Autodesk Inventor part; units mm, degrees
ref_plane "YZ Plane" through (0, 0, 0) normal (1, 0, 0) x (0, 1, 0)
ref_plane "XZ Plane" through (0, 0, 0) normal (0, 1, 0) x (-1, 0, 0)
ref_plane "XY Plane" through (0, 0, 0) normal (0, 0, 1) x (1, 0, 0)
sketch "Sketch17" plane through (0, 0, 0) normal (0, 0, 1) x (1, 0, 0)
  line L0 (-3.0888, 0.15) -> (-1.6743, 2.6)
  line L1 (-1.4145, 2.75) -> (1.4145, 2.75)
  line L2 (1.6743, 2.6) -> (3.0888, 0.15)
  line L3 (3.0888, -0.15) -> (1.6743, -2.6)
  line L4 (1.4145, -2.75) -> (-1.4145, -2.75)
  line L5 (-1.6743, -2.6) -> (-3.0888, -0.15)
  circle A0 centre (0, 0) radius 1.5
  arc A1 (-1.4145, 2.75) -> (-1.6743, 2.6) centre (-1.4145, 2.45) ccw
  arc A2 (1.6743, 2.6) -> (1.4145, 2.75) centre (1.4145, 2.45) ccw
  arc A3 (3.0888, -0.15) -> (3.0888, 0.15) centre (2.829, 0) ccw
  arc A4 (1.4145, -2.75) -> (1.6743, -2.6) centre (1.4145, -2.45) ccw
  arc A5 (-1.6743, -2.6) -> (-1.4145, -2.75) centre (-1.4145, -2.45) ccw
  arc A6 (-3.0888, 0.15) -> (-3.0888, -0.15) centre (-2.829, 0) ccw
  point P0 (-3.1754, 0)
  point P1 (-1.5877, 2.75)
  point P2 (1.5877, 2.75)
  point P3 (3.1754, 0)
  point P4 (1.5877, -2.75)
  point P5 (-1.5877, -2.75)
  dimension "d103" = 5.5
  dimension "d104" = 3
  dimension "d105" = 0.3
extrude "Extrusion14" add sketch "Sketch17" along normal blind 2.4
sketch "Sketch18" plane through (0, 0, 0) normal (0, 1, 0) x (-1, 0, 0)
  line L0 (-3.0888, 2.4) -> (-1.6743, 2.4)
  line L1 (-1.6743, 0) -> (-1.6743, 2.4)
  line L2 (-3.0888, 0) -> (-1.6743, 0)
  line L3 (-3.0888, 0) -> (-3.0888, 2.4)
  line L4 (-1.5, 2.4) -> (1.5, 2.4)
  line L5 (1.5, 0) -> (-1.5, 0)
  line L6 (1.6743, 2.4) -> (3.0888, 2.4)
  line L7 (3.0888, 0) -> (3.0888, 2.4)
  line L8 (1.6743, 0) -> (3.0888, 0)
  line L9 (1.6743, 0) -> (1.6743, 2.4)
  line L10 (0, 2.4) -> (0, 4.8692)
  line L11 (0, 4.8692) -> (0, -2.1161)
  line L12 (1.4145, 0) -> (1.6743, 0)
  line L13 (1.4145, 2.4) -> (1.6743, 2.4)
  line L14 (1.6743, 0) -> (1.6743, 2.4)
  line L15 (1.4145, 0) -> (1.6743, 0)
  line L16 (1.4145, 0) -> (1.4145, 2.4)
  line L17 (2.5888, 3.8507) -> (2.5888, -1.604) construction
  line L18 (4.0837, 1.5369) -> (4.0837, 3.518)
  line L19 (4.0837, 3.518) -> (2.5888, 3.518)
  line L20 (2.5888, 2.4) -> (2.5888, 3.518)
  line L21 (2.5888, 0) -> (4.2933, 0.9841)
  line L22 (4.2933, 0.9841) -> (4.2933, -0.6301)
  line L23 (4.2933, -0.6301) -> (2.5888, -0.6301)
  line L24 (2.5888, -0.6301) -> (2.5888, 0)
  line L25 (2.5888, 2.4) -> (4.0837, 1.5369)
  dimension "d110" = 30
  dimension "d111" = 30
  dimension "d115" = 0.5
revolve "Revolution1" cut sketch "Sketch18" angle 360 about axis through (0, 0, 4.8692) along (0, 0, -1) contours L20 L19 L18 L25 L7 L6 | L6 L7 L25 | L21 L7 L8 | L8 L7 L21 L22 L23 L24
thread "Thread3"
chamfer "Chaflán9" distance 0.2 angle 45 1 edges at (-1.5, 0, 2.4)
chamfer "Chaflán10" distance 0.2 angle 45 1 edges at (-1.5, 0, 0)
properties part number "CF-TCA-0001"
Geometry check sheet. Reference: the model listing, model coordinates, mm. Coordinates: 2 decimals unless noted, no trailing zeros. Order: outer loops, then holes, each group sorted by start corner. A loop starts at its lowest first (then second) coordinate and runs counter-clockwise, first axis right, second up.
Q1. Thickness scan on probe 1 along Y at (x, z) = (0, 1.4); probe 2 along Y at (x, z) = (-0.5, 1.85); probe 3 along X at (y, z) = (-0.7, 1.9). Record the ranges inside material, lowest first.
Reply:
probe 1: y = -2.75 to -1.5, 1.5 to 2.75
probe 2: y = -2.75 to -1.41, 1.41 to 2.75
probe 3: x = -2.77 to -1.33, 1.33 to 2.77
Q2. Draft check along X on faces 1 (the face through (2.39, -1.36, 1.18)), 2 (the face through (-1.5, -0.07, 1.19)), 3 (the face through (0, 2.75, 1)), 4 (the face through (-2.372, -1.392, 1.185)). Enter one of: released by +X, released by -X, zero draft, split by the parting line, or undercut.
Reply:
face 1: released by +X
face 2: undercut
face 3: zero draft
face 4: released by -X
Q3. Sectioned sample at A-A on x = 0. Record the cut outline in (y, z), and give its area (3 significant figures).
Reply:
outline: (-2.75, 0.09) - (-2.59, 0) - (-1.7, 0) - (-1.5, 0.2) - (-1.5, 2.2) - (-1.7, 2.4) - (-2.59, 2.4) - (-2.75, 2.31) - close; (1.5, 0.2) - (1.7, 0) - (2.59, 0) - (2.75, 0.09) - (2.75, 2.31) - (2.59, 2.4) - (1.7, 2.4) - (1.5, 2.2) - close
area: 5.89 mm2
Q4. Sectioned sample at B-B on z = 1.25. Record the cut outline in (x, y).
Reply:
outline: (-3.09, -0.15) - (-1.67, -2.6) arc R0.3 ccw to (-1.41, -2.75) - (1.41, -2.75) arc R0.3 ccw to (1.67, -2.6) - (3.09, -0.15) arc R0.3 ccw to (3.09, 0.15) - (1.67, 2.6) arc R0.3 ccw to (1.41, 2.75) - (-1.41, 2.75) arc R0.3 ccw to (-1.67, 2.6) - (-3.09, 0.15) arc R0.3 ccw to start; hole circle Ø3 at (0, 0)
Q5. Sectioned sample at C-C on y = 0. Record the cut outline in (x, z).
Reply:
outline: (-3.13, 0.31) - (-2.59, 0) - (-1.7, 0) - (-1.5, 0.2) - (-1.5, 2.2) - (-1.7, 2.4) - (-2.59, 2.4) - (-3.13, 2.09) - close; (1.5, 0.2) - (1.7, 0) - (2.59, 0) - (3.13, 0.31) - (3.13, 2.09) - (2.59, 2.4) - (1.7, 2.4) - (1.5, 2.2) - close
